```python
from build123d import *

# Parameters (mm, degrees)
SKETCH1_W          = 210
SKETCH1_H          = 210
BASE_DEPTH         = 16
CUT_EXTRUDE1_DEPTH = 12
FILLET1_R          = 5
FILLET2_R          = 5


with BuildPart() as part:
    # Sketch1 → Base (new body)
    with BuildSketch(Plane(origin=(0, 0, 0), x_dir=(1, 0, 0), z_dir=(0, 1, 0))):
        Rectangle(SKETCH1_W, SKETCH1_H)
    extrude(amount=BASE_DEPTH)

    # Sketch3 → Cut-Extrude1 (cut)
    with BuildSketch(Plane(origin=(0, 16, 0), x_dir=(1, 0, 0), z_dir=(0, 1, 0))):
        Polygon((-85, 95), (85, 95), (85, 85), (95, 85), (95, -85), (85, -85), (85, -95), (-85, -95), (-85, -85), (-95, -85), (-95, 85), (-85, 85), align=None)
    extrude(amount=-CUT_EXTRUDE1_DEPTH, mode=Mode.SUBTRACT)

    # Fillet1
    fillet1_edges = [part.edges().sort_by_distance(p)[0] for p in [
        (0, 0, 105),
        (-105, 0, 0),
        (0, 0, -105),
        (105, 0, 0),
    ]]
    fillet(fillet1_edges, radius=FILLET1_R)

    # Fillet2
    # the kernel refuses this fillet: 5 mm, written as the material it takes off along each edge
    with BuildSketch(Plane(origin=(100, 5, 100), x_dir=(1, 0, 0), z_dir=(0, 0, 1))) as fillet2_piece_1_section:
        Polygon((0, 0), (FILLET2_R, 0), (FILLET2_R, -FILLET2_R), (0, -FILLET2_R), align=None)
    fillet2_piece_1 = extrude(amount=FILLET2_R, mode=Mode.PRIVATE)
    fillet2_piece_1 = fillet2_piece_1 - Plane(origin=(100, 5, 100), x_dir=(-0.7071067811865475, 0.7071067811865475, 0), z_dir=(0, 0, 1)) * Sphere(FILLET2_R, mode=Mode.PRIVATE)
    add(fillet2_piece_1, mode=Mode.SUBTRACT)
    with BuildSketch(Plane(origin=(-100, 5, 100), x_dir=(-1, 0, 0), z_dir=(0, 0, 1))) as fillet2_piece_2_section:
        Polygon((0, 0), (FILLET2_R, 0), (FILLET2_R, FILLET2_R), (0, FILLET2_R), align=None)
    fillet2_piece_2 = extrude(amount=FILLET2_R, mode=Mode.PRIVATE)
    fillet2_piece_2 = fillet2_piece_2 - Plane(origin=(-100, 5, 100), x_dir=(0.7071067811865475, 0.7071067811865475, 0), z_dir=(0, 0, 1)) * Sphere(FILLET2_R, mode=Mode.PRIVATE)
    add(fillet2_piece_2, mode=Mode.SUBTRACT)
    with BuildSketch(Plane(origin=(100, 5, -100), x_dir=(0, 0, -1), z_dir=(1, 0, 0))) as fillet2_piece_3_section:
        Polygon((0, 0), (FILLET2_R, 0), (FILLET2_R, -FILLET2_R), (0, -FILLET2_R), align=None)
    fillet2_piece_3 = extrude(amount=FILLET2_R, mode=Mode.PRIVATE)
    fillet2_piece_3 = fillet2_piece_3 - Plane(origin=(100, 5, -100), x_dir=(0, 0.7071067811865475, 0.7071067811865475), z_dir=(1, 0, 0)) * Sphere(FILLET2_R, mode=Mode.PRIVATE)
    add(fillet2_piece_3, mode=Mode.SUBTRACT)
    with BuildSketch(Plane(origin=(-100, 5, -100), x_dir=(0, 0, -1), z_dir=(-1, 0, 0))) as fillet2_piece_4_section:
        Polygon((0, 0), (FILLET2_R, 0), (FILLET2_R, FILLET2_R), (0, FILLET2_R), align=None)
    fillet2_piece_4 = extrude(amount=FILLET2_R, mode=Mode.PRIVATE)
    fillet2_piece_4 = fillet2_piece_4 - Plane(origin=(-100, 5, -100), x_dir=(0, 0.7071067811865475, 0.7071067811865475), z_dir=(-1, 0, 0)) * Sphere(FILLET2_R, mode=Mode.PRIVATE)
    add(fillet2_piece_4, mode=Mode.SUBTRACT)
    with BuildSketch(Plane(origin=(105, 5, 105), x_dir=(-1, 0, 0), z_dir=(0, 1, 0)), Plane(origin=(105, 5, -105), x_dir=(0, 0, 1), z_dir=(0, 1, 0))) as fillet2_piece_5:
        with BuildLine():
            CenterArc((FILLET2_R, -FILLET2_R), FILLET2_R, 90, 90)
            Line((0, -FILLET2_R), (0, 0))
            Line((0, 0), (FILLET2_R, 0))
        make_face()
    extrude(amount=23.5, mode=Mode.SUBTRACT)
    with BuildSketch(Plane(origin=(-105, 5, 105), x_dir=(1, 0, 0), z_dir=(0, 1, 0)), Plane(origin=(-105, 5, -105), x_dir=(0, 0, 1), z_dir=(0, 1, 0))) as fillet2_piece_6:
        with BuildLine():
            CenterArc((FILLET2_R, FILLET2_R), FILLET2_R, 180, 90)
            Line((0, FILLET2_R), (0, 0))
            Line((0, 0), (FILLET2_R, 0))
        make_face()
    extrude(amount=23.5, mode=Mode.SUBTRACT)


solid = part.part
```
Could you check a few things on this model? Use its own coordinates, in mm. A direction names the side the tool comes from. Coordinates: 2 decimals unless noted, no trailing zeros. Loops run counter-clockwise (first coordinate to the right, second up) from the corner with the lowest first, then second, coordinate; pieces in that order, holes last.
1) Imagine slicing it at A-A (y = 10.5). List the corners of the cut face in (x, z) for me, and give its area (3 significant figures).
Reported:
outline: (-105, -100) arc R5 ccw to (-100, -105) - (100, -105) arc R5 ccw to (105, -100) - (105, 100) arc R5 ccw to (100, 105) - (-100, 105) arc R5 ccw to (-105, 100) - close; hole (-95, -85) - (-85, -85) - (-85, -95) - (85, -95) - (85, -85) - (95, -85) - (95, 85) - (85, 85) - (85, 95) - (-85, 95) - (-85, 85) - (-95, 85) - close
area: 8,380 mm2
2) Imagine slicing it at C-C (z = -51.5). List the corners of the cut face in (x, y) for me.
Reported:
outline: (-105, 5) arc R5 ccw to (-100, 0) - (100, 0) arc R5 ccw to (105, 5) - (105, 16) - (95, 16) - (95, 4) - (-95, 4) - (-95, 16) - (-105, 16) - close
3) Will these pins go through, and if not, where does the flat tip stop? pin 1 Ø10 at (x, z) = (-5, 61.5) entering from +Y; pin 2 Ø6 at (x, y) = (65, 3) entering from -Z.
Reported:
pin 1: stops at y = 4
pin 2: stops at z = -105
4) Imagine slicing it at B-B (x = -21). List the corners of the cut face in (y, z) for me.
Reported:
outline: (0, -100) arc R5 ccw to (5, -105) - (16, -105) - (16, -95) - (4, -95) - (4, 95) - (16, 95) - (16, 105) - (5, 105) arc R5 ccw to (0, 100) - close
5) Which directions (+Z, -Z, +X, -X, +Y, -Y) give clear straight access to the entire face, cutting with the end or side of a thin tool? Please do faces 5 (the face through (1, 2, 104)), 6 (the face through (-95, 10, 1)).
Reported:
face 5: +Z, +X, -X, -Y
face 6: +Y
6) Thinking about a two-plate mould opening in Z: for faces 1 (the face through (-85, 10, 90)), 2 (the face through (1, 2, -104)), 3 (the face through (1, 10, 95)), 4 (the face through (-1, 10, 105)), which applies, released by +Z, released by -Z, zero draft, split by the parting line, or undercut?
Reported:
face 1: undercut
face 2: released by -Z
face 3: undercut
face 4: released by +Z
7) Please list where these lines run through material, in increasing order: line 1 along Z through (x, y) = (83, 12.75); line 2 along Z through (x, y) = (91, 15.25).
Reported:
line 1: z = -105 to -95, 95 to 105
line 2: z = -105 to -85, 85 to 105
